Can you work these out from the model? Positions are in its coordinate system, mm. A direction names the side the tool comes from. Give positions to 0.01 mm unless a question says otherwise; leave off trailing zeros. Order: outer loops, then holes, each group sorted by start corner. A loop starts at its lowest first (then second) coordinate and runs counter-clockwise, first axis right, second up. Notation, with made-up numbers: (81, -37) - (103, -37) arc R17 cw to (103, -20) - close; hole circle Ø2 at (77, 25.25). An arc over 180 degrees is marked (long way). Use one line per item in the form item = value. Start each with the question number.
1) Which directions (+Z, -Z, +X, -X, +Y, -Y) give clear straight access to the entire face, cutting with the end or side of a thin tool? Please do faces 1 (the cylindrical face through (-23.028, -7.225, 32.015)), 2 (the flat face through (0, 0, 41.3)), 3 (the flat face through (-26.5, 0, 31)), 4 (the cylindrical face through (24.7, 0.1, 34.3)).
2) Suppose I cut it at B-B, the plane z = 7. Write out the boundary of the cut face in (x, y), and give its area (3 significant figures).
3) Suppose I cut it at A-A, the plane y = 0. Write out the boundary of the cut face in (x, z), and give its area (3 significant figures).
4) Suppose I cut it at D-D, the plane z = 23.85. Write out the boundary of the cut face in (x, y).
5) Please list where these lines run through material, in increasing order: probe 1 along Y at (x, z) = (-23.55, 31.3); probe 2 along X at (y, z) = (-2, 12); probe 3 along X at (y, z) = (1, 27).
6) For pin 1 (1.6 mm diameter, centred on y = 7.5, z = 31.5, fed in from -X); pin 2 (1.2 mm diameter, centred on y = 0, z = 38.75, fed in from -X); pin 3 (1.5 mm diameter, centred on y = 3.5, z = 10.5, fed in from -X), each with a flat end and sliding along its axis, tell me the tip position at first contact or that it passes through.
7) Suppose I cut it at C-C, the plane y = 7.45. Write out the boundary of the cut face in (x, z), and give its area (3 significant figures).
8) We'd pull the mould along Y, two halves only. Please class faces 5 (the flat face through (-21, 7, 31)), 6 (the flat face through (27.9, 0, 31)), 7 (the flat face through (0, 10.5, 20)): released by +Y, released by -Y, zero draft, split by the parting line, or undercut.
```python
from build123d import *

# Parameters (mm, degrees)
SKETCH_1_W          = 43
SKETCH_1_H          = 21
EXTRUDE_1_DEPTH     = 41.3
SKETCH_2_R          = 3
EXTRUDE_2_DEPTH     = 6.4
SKETCH_3_R          = 10.35
EXTRUDE_3_DEPTH     = 3.5
SKETCH_4_R          = 6
EXTRUDE_4_DEPTH     = 1.5
SKETCH_5_R          = 0.75
CUT_EXTRUDE_1_DEPTH = 4


with BuildPart() as part:
    # 草图1 → 凸台-拉伸1 (new body)
    with BuildSketch(Plane.XY):
        Rectangle(SKETCH_1_W, SKETCH_1_H)
    extrude(amount=EXTRUDE_1_DEPTH)

    # 草图2 → 凸台-拉伸2 (add)
    with BuildSketch(Plane(origin=(21.5, 0, 0), x_dir=(0, 0, -1), z_dir=(1, 0, 0))):
        with Locations((-31.3, 0)):
            Circle(SKETCH_2_R)
    extrude(amount=EXTRUDE_2_DEPTH)

    # 草图3 → 凸台-拉伸3 (add)
    with BuildSketch(Plane.ZY.offset(21.5)):
        with Locations((31.3, 0)):
            Circle(SKETCH_3_R)
    extrude(amount=EXTRUDE_3_DEPTH)

    # 草图4 → 凸台-拉伸4 (add)
    with BuildSketch(Plane.ZY.offset(25)):
        with Locations((31.3, 0)):
            Circle(SKETCH_4_R)
    extrude(amount=EXTRUDE_4_DEPTH)

    # 草图5 → 切除-拉伸1 (cut)
    with BuildSketch(Plane.ZY.offset(25)):
        with Locations((38.75, 0)):
            Circle(SKETCH_5_R)
        with Locations((31.3, -7.45)):
            Circle(SKETCH_5_R)
        with Locations((23.85, 0)):
            Circle(SKETCH_5_R)
        with Locations((31.3, 7.45)):
            Circle(SKETCH_5_R)
    extrude(amount=-CUT_EXTRUDE_1_DEPTH, mode=Mode.SUBTRACT)


solid = part.part
```
Result sheet:
q1.face_1 = -X
q1.face_2 = +Z, +X, +Y, -Y
q1.face_3 = +Z, -Z, -X, +Y, -Y
q1.face_4 = +X
q2.outline = (-21.5, -10.5) - (21.5, -10.5) - (21.5, 10.5) - (-21.5, 10.5) - close
q2.area = 903 mm²
q3.outline = (-26.5, 25.3) - (-25, 25.3) - (-25, 24.6) - (-21, 24.6) - (-21, 23.1) - (-25, 23.1) - (-25, 20.95) - (-21.5, 20.95) - (-21.5, 0) - (21.5, 0) - (21.5, 28.3) - (27.9, 28.3) - (27.9, 34.3) - (21.5, 34.3) - (21.5, 41.3) - (-21.5, 41.3) - (-21.5, 41.65) - (-25, 41.65) - (-25, 39.5) - (-21, 39.5) - (-21, 38) - (-25, 38) - (-25, 37.3) - (-26.5, 37.3) - close
q3.area = 1,890 mm²
q4.outline = (-25, -7.18) - (-21.5, -7.18) - (-21.5, -10.5) - (21.5, -10.5) - (21.5, 10.5) - (-21.5, 10.5) - (-21.5, 7.18) - (-25, 7.18) - (-25, 0.75) - (-21, 0.75) - (-21, -0.75) - (-25, -0.75) - close
q5.probe_1 = -10.35 to -8.2, -6.7 to 6.7, 8.2 to 10.35
q5.probe_2 = -21.5 to 21.5
q5.probe_3 = -26.5 to 21.5
q6.pin_1 = -25
q6.pin_2 = -21
q6.pin_3 = -21.5
q7.outline = (-25, 24.12) - (-21.5, 24.12) - (-21.5, 0) - (21.5, 0) - (21.5, 41.3) - (-21.5, 41.3) - (-21.5, 38.48) - (-25, 38.48) - (-25, 32.05) - (-21, 32.05) - (-21, 30.55) - (-25, 30.55) - close
q7.area = 1,820 mm²
q8.face_5 = undercut
q8.face_6 = zero draft
q8.face_7 = released by +Y
